The model under review builds one solid part; all positions refer to its coordinate system, in mm. Give positions to 0.01 mm unless a question says otherwise; leave off trailing zeros. Order: outer loops, then holes, each group sorted by start corner. A loop starts at its lowest first (then second) coordinate and runs counter-clockwise, first axis right, second up. Notation, with made-up numbers: (52.5, 3) - (59.5, 3) arc R19 ccw to (59.5, 39) - close; hole circle Ø3 at (49.25, 4). An arc over 180 degrees is marked (long way). Answer as CSV lines item,"result". Start each with the question number.
Autodesk Inventor part; units mm, degrees
ref_plane "YZ Plane" through (0, 0, 0) normal (1, 0, 0) x (0, 1, 0)
ref_plane "XZ Plane" through (0, 0, 0) normal (0, 1, 0) x (-1, 0, 0)
ref_plane "XY Plane" through (0, 0, 0) normal (0, 0, 1) x (1, 0, 0)
sketch "Sketch1" plane through (0, 0, 0) normal (0, 0, 1) x (1, 0, 0)
  line L0 (4, -2.3094) -> (0, -4.6188)
  line L1 (0, -4.6188) -> (-4, -2.3094)
  line L2 (-4, -2.3094) -> (-4, 2.3094)
  line L3 (-4, 2.3094) -> (0, 4.6188)
  line L4 (0, 4.6188) -> (4, 2.3094)
  line L5 (4, 2.3094) -> (4, -2.3094)
  circle A0 centre (0, 0) radius 2.5
  dimension "d0" = 8
  dimension "d1" = 5
extrude "Extrusion1" add sketch "Sketch1" along normal blind 5
sketch "Sketch4" plane through (0, 0, 0) normal (1, 0, 0) x (0, 1, 0)
  line L0 (-4.6188, 0) -> (-2.3094, 0)
  line L1 (-4.6188, 0) -> (-4.6188, 5)
  line L2 (-2.3094, 5) -> (-4.6188, 5)
  line L3 (-2.3094, 0) -> (-2.3094, 5)
  line L4 (2.3094, 0) -> (4.6188, 0)
  line L5 (2.3094, 0) -> (2.3094, 5)
  line L6 (4.6188, 5) -> (2.3094, 5)
  line L7 (4.6188, 0) -> (4.6188, 5)
  arc A0 (-3.1388, 5) -> (-3.854, 3.9517) centre (-0.7691, 2.615) ccw
  arc A1 (-3.854, 3.9517) -> (-4.6188, 3.6047) centre (-1.2465, -2.8098) ccw
  line L8 (0, 0) -> (0, 9.301) construction
  arc A2 (3.7221, 0) -> (4.6188, 0.5597) centre (0, 6.9619) ccw
  arc A3 (-4.6188, 0.4688) -> (-3.8763, 0) centre (0, 6.9619) ccw
revolve "Revolution3" cut sketch "Sketch4" angle 360 about axis through (0, 0, 0) along (0, 0, 1) contours L1 A3 L0 | L1 L2 A0 A1
thread "Thread1"
properties part number "M5 Nylock"
Item 1: Take a section at A-A on z = 1.3. Write out the cut boundary in (x, y).
Item 2: Clearance check with flat-ended pins moving along their axes: pin 1 (1.5 mm diameter, centred on x = -1, z = 3, fed in from -Y); pin 2 (3 mm diameter, centred on x = -1, z = 3.5, fed in from +Y); pin 3 (1.5 mm diameter, centred on x = -1.5, z = 3.5, fed in from -Y); pin 4 (4 mm diameter, centred on x = 0, y = 0, fed in from +Z). State where each tip first meets the part, or that it passes through.
Item 3: For line 1 along X through (y, z) = (-1.5, 0.5); line 2 along Y through (x, z) = (1.5, 1.25); line 3 along X through (y, z) = (-0.5, 0.6), list the stretches that pass through material, from the lowest coordinate up.
Data:
1,outline,"(-4, -2.31) - (0, -4.62) - (4, -2.31) - (4, 2.31) - (0, 4.62) - (-4, 2.31) - close; hole circle Ø5 at (0, 0)"
2,pin 1,"stops at y = -4.47"
2,pin 2,"stops at y = 4.62"
2,pin 3,"stops at y = -4.19"
2,pin 4,"passes through"
3,line 1,"x = -4 to -2, 2 to 4"
3,line 2,"y = -3.75 to -2, 2 to 3.75"
3,line 3,"x = -4 to -2.45, 2.45 to 4"
